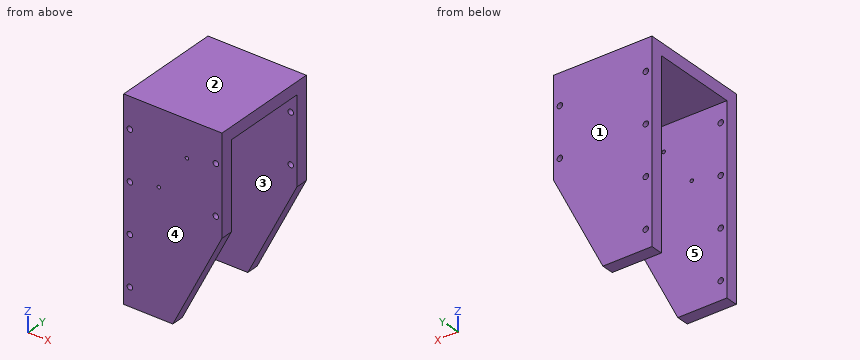
from build123d import *

# Parameters (mm, degrees)
SALIENTE_EXTRUIR1_DEPTH = 10
CROQUIS2_W              = 80
CROQUIS2_H              = 10
SALIENTE_EXTRUIR2_DEPTH = 70
SALIENTE_EXTRUIR3_DEPTH = 10
CROQUIS4_R              = 2.25
CORTAR_EXTRUIR1_DEPTH   = 201.249843945
CORTAR_EXTRUIR2_REACH   = 202.25
CROQUIS5_R              = 1.4


with BuildPart() as part:
    # Croquis1 → Saliente-Extruir1 (new body)
    with BuildSketch(Plane(origin=(0, 0, 0), x_dir=(1, 0, 0), z_dir=(0, 1, 0))):
        Polygon((0, 0), (0, 80), (-40, 160), (-80, 160), (-80, 0), align=None)
    extrude(amount=SALIENTE_EXTRUIR1_DEPTH)

    # Croquis2 → Saliente-Extruir2 (add)
    with BuildSketch(Plane(origin=(0, 10, 0), x_dir=(1, 0, 0), z_dir=(0, 1, 0))):
        with Locations((-40, 5)):
            Rectangle(CROQUIS2_W, CROQUIS2_H)
    extrude(amount=SALIENTE_EXTRUIR2_DEPTH)

    # Croquis3 → Saliente-Extruir3 (add)
    with BuildSketch(Plane(origin=(0, 80, 0), x_dir=(1, 0, 0), z_dir=(0, 1, 0))):
        Polygon((-80, 0), (0, 0), (0, 80), (-40, 160), (-80, 160), align=None)
    extrude(amount=SALIENTE_EXTRUIR3_DEPTH)

    # Croquis4 → Cortar-Extruir1 (cut, through all)
    with BuildSketch(Plane(origin=(0, 90, 0), x_dir=(1, 0, 0), z_dir=(0, 1, 0))):
        with Locations(Location((-75, 25, 0), (0, 0, 270))):
            Circle(CROQUIS4_R)
        with Locations(Location((-5, 25, 0), (0, 0, 270))):
            Circle(CROQUIS4_R)
        with Locations(Location((-5, 65, 0), (0, 0, 270))):
            Circle(CROQUIS4_R)
        with Locations(Location((-75, 65, 0), (0, 0, 270))):
            Circle(CROQUIS4_R)
        with Locations(Location((-75, 145, 0), (0, 0, 270))):
            Circle(CROQUIS4_R)
        with Locations(Location((-75, 105, 0), (0, 0, 270))):
            Circle(CROQUIS4_R)
    extrude(amount=-CORTAR_EXTRUIR1_DEPTH, mode=Mode.SUBTRACT)

    # Croquis5 → Cortar-Extruir2 (cut, up to next)
    with BuildSketch(Plane.XZ, mode=Mode.PRIVATE) as cortar_extruir2_sk1:
        with Locations(Location((-28.57, -29.76, 0), (0, 0, 270))):
            Circle(CROQUIS5_R)
    cortar_extruir2_tool1 = extrude(cortar_extruir2_sk1.sketch, amount=-CORTAR_EXTRUIR2_REACH, mode=Mode.PRIVATE) & part.part
    # Croquis5 → Cortar-Extruir2 (cut, up to next)
    with BuildSketch(Plane.XZ, mode=Mode.PRIVATE) as cortar_extruir2_sk2:
        with Locations(Location((-51.43, -60.24, 0), (0, 0, 270))):
            Circle(CROQUIS5_R)
    cortar_extruir2_tool2 = extrude(cortar_extruir2_sk2.sketch, amount=-CORTAR_EXTRUIR2_REACH, mode=Mode.PRIVATE) & part.part
    add(cortar_extruir2_tool1.solids().sort_by_distance((-28.57, 0, -29.76))[0], mode=Mode.SUBTRACT)
    add(cortar_extruir2_tool2.solids().sort_by_distance((-51.43, 0, -60.24))[0], mode=Mode.SUBTRACT)


solid = part.part
Geometry: final body of the model. Coordinates: model frame, mm. Face numbers are marked on the shaded views. A direction names the side the tool comes from. Round coordinates to 2 decimals unless told otherwise and drop trailing zeros. Loops run counter-clockwise (first coordinate to the right, second up) from the corner with the lowest first, then second, coordinate; pieces in that order, holes last. Notation, with made-up numbers: (33.5, -17) - (76.5, -17) arc R20 cw to (76.5, 11) - close; hole circle Ø2 at (31.5, 77). An arc over 180 degrees is marked (long way). Write each question's results on one line, items separated by ' | '. Start each with the question number.
1) Cut plane A-A on z = -93.5. Return loops of the section in (x, y).
2) Line query: probe 1 along Y at (x, z) = (-62, -153); probe 2 along Z at (x, y) = (-42.5, 41); probe 3 along X at (y, z) = (6.5, -145). Output: solid intervals per line, ascending. Write a range as [from, to].
3) Access query for the marked faces 4 and 5. Directions: +Z, -Z, +X, -X, +Y, -Y. A direction counts if a zero-diameter tool reaches every point of the face in a straight line with its end or side. Return the directions, or none.
4) Cut plane C-C on z = -65. Return loops of the section in (x, y).
5) First-contact query: P1, Ø1, axis at x = -61.5, y = 69.5, coming from the +Z side; P2, Ø3.5, axis at x = -75, z = -145, coming from the -Y side; P3, Ø1.7, axis at x = -51.43, z = -60.24, coming from the -Y side; P4, Ø2, axis at x = -27, y = 69, coming from the -Z side. Flat tips, straight axial feed; report the tip coordinate or a pass-through.
6) Cut plane D-D on y = 84. Return loops of the section in (x, z).
7) Cut plane B-B on x = -5. Return loops of the section in (y, z), then the cut area to 3 significant figures.
8) Mould query, pull axis Y, two halves, no side actions, for the marked faces 1, 2 and 3. Classes: released by +Y, released by -Y, zero draft, split by the parting line, or undercut.
Verdict:
1) outline: (-80, 0) - (-6.75, 0) - (-6.75, 10) - (-80, 10) - close; (-80, 80) - (-6.75, 80) - (-6.75, 90) - (-80, 90) - close
2) probe 1: y = [0, 10], [80, 90] | probe 2: z = [-10, 0] | probe 3: x = [-80, -77.25], [-72.75, -32.5]
3) face 4: +Z, -Z, +X, -X, -Y | face 5: -Z, +X, -X
4) outline: (-80, 0) - (-77.25, 0) - (-77.25, 10) - (-80, 10) - close; (-80, 80) - (-77.25, 80) - (-77.25, 90) - (-80, 90) - close; (-72.75, 0) - (-7.25, 0) - (-7.25, 10) - (-72.75, 10) - close; (-72.75, 80) - (-7.25, 80) - (-7.25, 90) - (-72.75, 90) - close; (-2.75, 0) - (0, 0) - (0, 10) - (-2.75, 10) - close; (-2.75, 80) - (0, 80) - (0, 90) - (-2.75, 90) - close
5) P1: stops at z = 0 | P2: passes through | P3: stops at y = 80 | P4: stops at z = -10
6) outline: (-80, -160) - (-40, -160) - (0, -80) - (0, 0) - (-80, 0) - close; hole circle Ø4.5 at (-75, -145); hole circle Ø4.5 at (-75, -105); hole circle Ø4.5 at (-75, -65); hole circle Ø4.5 at (-75, -25); hole circle Ø4.5 at (-5, -65); hole circle Ø4.5 at (-5, -25)
7) outline: (0, -90) - (10, -90) - (10, -67.25) - (0, -67.25) - close; (0, -62.75) - (10, -62.75) - (10, -27.25) - (0, -27.25) - close; (0, -22.75) - (10, -22.75) - (10, -10) - (80, -10) - (80, -22.75) - (90, -22.75) - (90, 0) - (0, 0) - close; (80, -90) - (90, -90) - (90, -67.25) - (80, -67.25) - close; (80, -62.75) - (90, -62.75) - (90, -27.25) - (80, -27.25) - close | area: 2,320 mm2
8) face 1: released by +Y | face 2: zero draft | face 3: undercut
